```python
from build123d import *


with BuildPart() as part:
    # Sketch 3 → Revolve 2 (revolve)
    with BuildSketch(Plane(origin=(0, 0, 0), x_dir=(1, 0, 0), z_dir=(0, 1, 0)), mode=Mode.PRIVATE) as revolve_2_sk:
        with BuildLine():
            Line((-10, 15), (10, 15))
            Line((10, 15), (10, 9.660444431))
            ThreePointArc((10, 9.660444431), (9.414213562, 8.246230869), (8, 7.660444431))
            Line((8, 7.660444431), (6.427876097, 7.660444431))
            ThreePointArc((6.427876097, 7.660444431), (0, 10), (-6.427876097, 7.660444431))
            Line((-6.427876097, 7.660444431), (-8, 7.660444431))
            ThreePointArc((-8, 7.660444431), (-9.414213562, 8.246230869), (-10, 9.660444431))
            Line((-10, 9.660444431), (-10, 15))
        make_face()
    revolve(revolve_2_sk.sketch.rotate(Axis((115, 0, 57.074015866), (0, 0, -1)), 180), axis=Axis((115, 0, 57.074015866), (0, 0, -1)))


solid = part.part
```
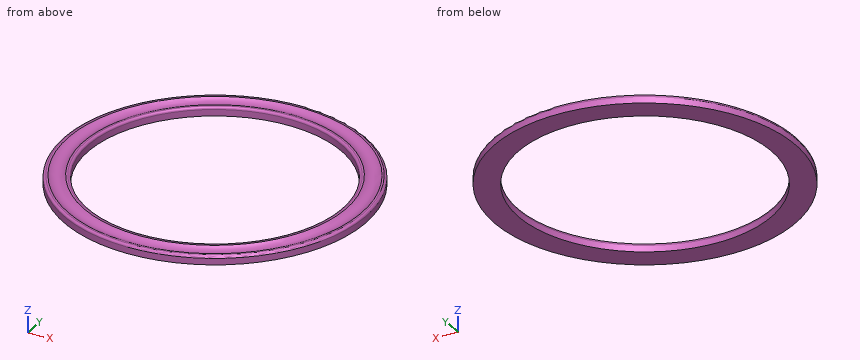
Here's how the part is built. I have some questions about the finished solid (model axes, mm). Coordinates: 2 decimals unless noted, no trailing zeros. Loops run counter-clockwise (first coordinate to the right, second up) from the corner with the lowest first, then second, coordinate; pieces in that order, holes last. Notation, with made-up numbers: (79.5, 30.25) - (101.5, 30.25) arc R33 cw to (101.5, 69.25) - close; hole circle Ø2 at (-38, -25). An arc over 180 degrees is marked (long way). Return JSON: item names as keys, results as strings. Group by question number.
Item 1: If we section it at C-C on z = -11.5: Write out the boundary of the cut face in (x, y).
Item 2: Will this pin go through, and if not, where does the flat tip stop? P1, Ø4, axis at y = -24, z = -12, coming from the +X side.
Item 3: If we section it at A-A on x = 115: Write out the boundary of the cut face in (y, z).
Item 4: I need wall thicknesses on line 1 (X direction, y = 79, z = -8.25); line 2 (Y direction, x = 115, z = -11); line 3 (X direction, y = 41.5, z = -9). Which ranges of each line are inside material? Lowest first, please. Write a range as from..to.
Item 5: If we section it at B-B on y = 0: Write out the boundary of the cut face in (x, z).
Calculated:
{
 "1": {"outline": "circle Ø250 at (115, 0); hole circle Ø210 at (115, 0)"},
 "2": {"P1": "stops at x = 238.05"},
 "3": {"outline": "(-125, -15) - (-105, -15) - (-105, -9.66) arc R2 ccw to (-107, -7.66) - (-108.57, -7.66) arc R10 cw to (-121.43, -7.66) - (-123, -7.66) arc R2 ccw to (-125, -9.66) - close; (105, -15) - (125, -15) - (125, -9.66) arc R2 ccw to (123, -7.66) - (121.43, -7.66) arc R10 cw to (108.57, -7.66) - (107, -7.66) arc R2 ccw to (105, -9.66) - close"},
 "4": {"line 1": "x = 18.88..23.81, 39.39..44.95, 185.05..190.61, 206.19..211.12", "line 2": "y = -125..-105, 105..125", "line 3": "x = -2.79..3.09, 12.44..18.43, 211.57..217.56, 226.91..232.79"},
 "5": {"outline": "(-10, -15) - (10, -15) - (10, -9.66) arc R2 ccw to (8, -7.66) - (6.43, -7.66) arc R10 cw to (-6.43, -7.66) - (-8, -7.66) arc R2 ccw to (-10, -9.66) - close; (220, -15) - (240, -15) - (240, -9.66) arc R2 ccw to (238, -7.66) - (236.43, -7.66) arc R10 cw to (223.57, -7.66) - (222, -7.66) arc R2 ccw to (220, -9.66) - close"}
}
